```python
from build123d import *

# Parameters (mm, degrees)
ESQUISSE1_W             = 16
ESQUISSE1_H             = 8
ESQUISSE1_R             = 3
BOSS_EXTRU_1_DEPTH      = 16
ESQUISSE2_R             = 2.5
ENL_V_MAT_EXTRU_1_DEPTH = 9
CHANFREIN1_SIZE         = 0.5
CONG_1_R                = 0.5


with BuildPart() as part:
    # Esquisse1 → Boss.-Extru.1 (new body)
    with BuildSketch(Plane.XY):
        with Locations((8, 4)):
            Rectangle(ESQUISSE1_W, ESQUISSE1_H)
        with Locations((12, 4)):
            Circle(ESQUISSE1_R, mode=Mode.SUBTRACT)
    extrude(amount=BOSS_EXTRU_1_DEPTH)

    # Esquisse2 → Enlèv. mat.-Extru.1 (cut, through all)
    with BuildSketch(Plane(origin=(0, 8, 0), x_dir=(1, 0, 0), z_dir=(0, 1, 0))):
        with Locations((4, -8)):
            Circle(ESQUISSE2_R)
    extrude(amount=-ENL_V_MAT_EXTRU_1_DEPTH, mode=Mode.SUBTRACT)

    # Chanfrein1
    chanfrein1_edges = [part.edges().sort_by_distance(p)[0] for p in [
        (1.5, 0, 8),
        (1.5, 8, 8),
    ]]
    chamfer(chanfrein1_edges, length=CHANFREIN1_SIZE)

    # Congé1
    cong_1_edges = [part.edges().sort_by_distance(p)[0] for p in [
        (9, 4, 0),
        (9, 4, 16),
    ]]
    fillet(cong_1_edges, radius=CONG_1_R)


solid = part.part
```
Read the model definition and answer for the solid it produces. Units are mm, in the model's axes. Give positions to 0.01 mm unless a question says otherwise; leave off trailing zeros. Order: outer loops, then holes, each group sorted by start corner. A loop starts at its lowest first (then second) coordinate and runs counter-clockwise, first axis right, second up.
(1) Find section B-B (z = 8). Give the vertices of the cut face in (x, y).
(2) Given pin 1 (3 mm diameter, centred on x = 4, z = 8, fed in from -Y) (3 decimals), flat-ended and moving along its own axis, determine where the tip first touches the part or whether it passes through.
(3) Find section C-C (y = 4). Give the vertices of the cut face in (x, z), plus the area to 3 significant figures.
(4) Straight lines are drawn through the part: L1, parallel to X at y = 5.5, z = 8; L2, parallel to X at y = 4.75, z = 6.5; L3, parallel to Z at x = 4, y = 5. For each, find the intervals that lie inside material, in ascending order.
(5) Find section A-A (x = 12). Give the vertices of the cut face in (y, z).
(6) Find section D-D (z = 1.5). Give the vertices of the cut face in (x, y).
(7) For a pull along X with two mould halves and no side action, classify faces 1 (the cylindrical face through (5.15, 4.05, 10.22)), 2 (the flat face through (8, 8, 8)), 3 (the flat face through (0, 4, 8)) as released by +X, released by -X, zero draft, split by the parting line, or undercut.
Result sheet:
1. outline: (0, 0) - (1, 0) - (1.5, 0.5) - (1.5, 7.5) - (1, 8) - (0, 8) - close; (6.5, 0.5) - (7, 0) - (16, 0) - (16, 8) - (7, 8) - (6.5, 7.5) - close; hole circle Ø6 at (12, 4)
2. pin 1: passes through
3. outline: (0, 0) - (8.5, 0) arc R0.5 ccw to (9, 0.5) - (9, 15.5) arc R0.5 ccw to (8.5, 16) - (0, 16) - close; (15, 0.5) arc R0.5 ccw to (15.5, 0) - (16, 0) - (16, 16) - (15.5, 16) arc R0.5 ccw to (15, 15.5) - close; hole circle Ø5 at (4, 8)
3. area: 140 mm2
4. L1: x = 0 to 1.5, 6.5 to 9.4, 14.6 to 16
4. L2: x = 0 to 2, 6 to 9.1, 14.9 to 16
4. L3: z = 0 to 5.5, 10.5 to 16
5. outline: (0, 0) - (0.5, 0) arc R0.5 ccw to (1, 0.5) - (1, 15.5) arc R0.5 ccw to (0.5, 16) - (0, 16) - close; (7, 0.5) arc R0.5 ccw to (7.5, 0) - (8, 0) - (8, 16) - (7.5, 16) arc R0.5 ccw to (7, 15.5) - close
6. outline: (0, 0) - (16, 0) - (16, 8) - (0, 8) - close; hole circle Ø6 at (12, 4)
7. face 1: undercut
7. face 2: zero draft
7. face 3: released by -X
